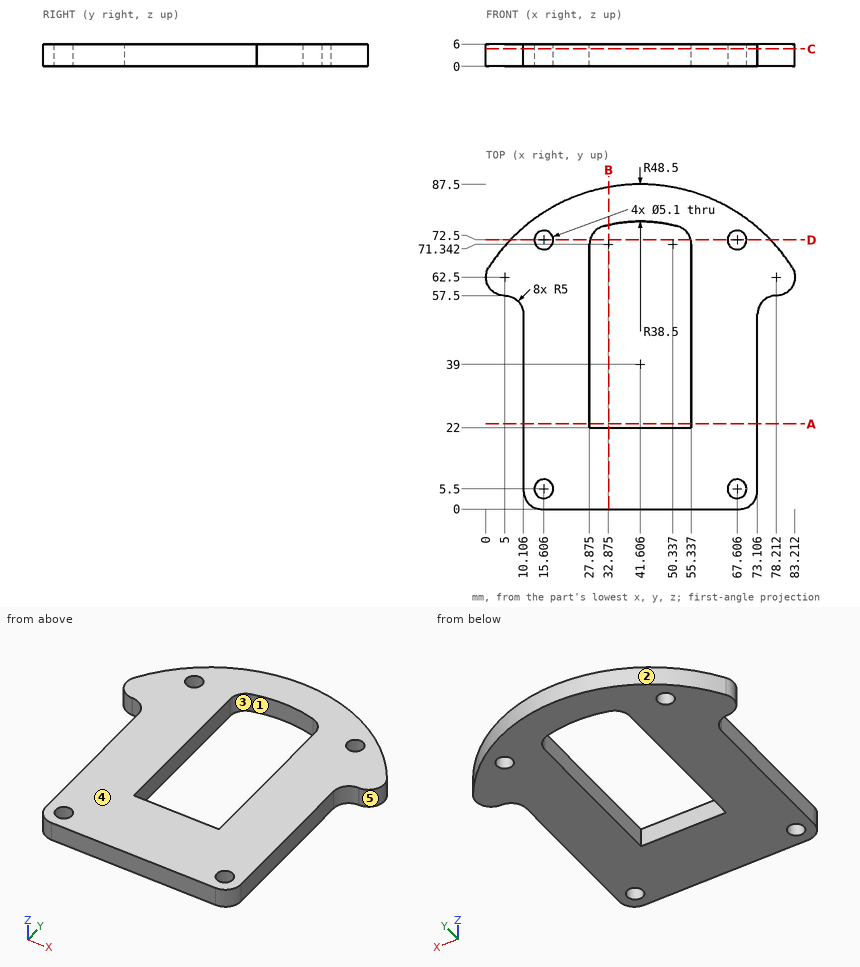
Can you work these out from the drawing? Everything is in mm from the part's minimum corner. A direction names the side the tool comes from. Coordinates: 2 decimals unless noted, no trailing zeros. Loops run counter-clockwise (first coordinate to the right, second up) from the corner with the lowest first, then second, coordinate; pieces in that order, holes last.
1) Imagine slicing it at B-B on x = 33. List the corners of the cut face in (y, z) for me.
2) I need wall thicknesses on probe 1 along X at (y, z) = (26.5, 1.7) (1 decimal); probe 2 along Y at (x, z) = (69, 4.65) (1 decimal); probe 3 along X at (y, z) = (72.5, 4.6) (1 decimal). Which ranges of each line are inside material? Lowest first, please.
3) Thinking about a two-plate mould opening in X: for the marked faces 3, 4 and 5, which applies, pulls with the +X half, pulls with the -X half, needs draft (parallel to the pull), parting line crosses it, or undercut?
4) Imagine slicing it at C-C on z = 4.7. State how many separate pieces and enclosed holes the cut face has, plus the area to 3 significant figures.
5) Imagine slicing it at D-D on y = 72.5. List the corners of the cut face in (x, z) for me (1 decimal).
6) Imagine slicing it at A-A on y = 23. List the corners of the cut face in (x, z) for me (1 decimal), plus the area to 3 significant figures.
7) Which directions (+Z, -Z, +X, -X, +Y, -Y) give clear straight access to the entire face, cutting with the end or side of a thin tool? Please do the marked faces 1 and 2.
8) For pin 1 (2 mm diameter, centred on x = 64, z = 1, fed in from -Y); pin 2 (1 mm diameter, centred on y = 22.5, z = 0.5, fed in from +X); pin 3 (1 mm diameter, centred on y = 43, z = 1.5, fed in from -X), each with a flat end and sliding along its axis, tell me the tip position at first contact or that it passes through.
Completed:
1. outline: (0, 0) - (22, 0) - (22, 6) - (0, 6) - close; (76.53, 0) - (86.73, 0) - (86.73, 6) - (76.53, 6) - close
2. probe 1: x = 10.1 to 27.9, 55.3 to 73.1
2. probe 2: y = 0.1 to 3.4, 7.6 to 70.4, 74.6 to 79
2. probe 3: x = 6.5 to 13.1, 18.2 to 28, 55.2 to 65.1, 70.2 to 76.7
3. face 3: undercut
3. face 4: needs draft
3. face 5: pulls with the +X half
4. separate pieces: 1
4. enclosed holes: 5
4. area: 3,960 mm2
5. outline: (6.5, 0) - (13.1, 0) - (13.1, 6) - (6.5, 6) - close; (18.2, 0) - (28, 0) - (28, 6) - (18.2, 6) - close; (55.2, 0) - (65.1, 0) - (65.1, 6) - (55.2, 6) - close; (70.2, 0) - (76.7, 0) - (76.7, 6) - (70.2, 6) - close
6. outline: (10.1, 0) - (27.9, 0) - (27.9, 6) - (10.1, 6) - close; (55.3, 0) - (73.1, 0) - (73.1, 6) - (55.3, 6) - close
6. area: 213 mm2
7. face 1: +Z, -Z
7. face 2: +Z, -Z, +Y
8. pin 1: stops at y = 0
8. pin 2: stops at x = 73.11
8. pin 3: stops at x = 10.11
